Geometry check sheet. Reference: the model listing, model coordinates, mm. A direction names the side the tool comes from. Give positions to 0.01 mm unless a question says otherwise; leave off trailing zeros. Loops run counter-clockwise (first coordinate to the right, second up) from the corner with the lowest first, then second, coordinate; pieces in that order, holes last. Notation, with made-up numbers: (2.25, 52) -> (28.25, 52) arc R22 ccw to (28.25, 87) -> close; hole circle Ø3 at (-35.5, -4). An arc over 180 degrees is marked (long way). Write item = value, one per line.
```python
from build123d import *

# Parameters (mm, degrees)
SKETCH_1_W                 = 240
SKETCH_1_H                 = 100
EXTRUDE_1_DEPTH            = 6
SKETCH_2_R                 = 1.55
CUT_EXTRUDE_1_DEPTH        = 261.069221555
SKETCH_3_W                 = 60
SKETCH_3_H                 = 15
CUT_EXTRUDE_2_DEPTH        = 261.069221555
SKETCH_4_W                 = 30
SKETCH_4_H                 = 80
CUT_EXTRUDE_3_DEPTH        = 261.069221555
SKETCH_5_R                 = 3
CUT_EXTRUDE_4_DEPTH        = 3
EXTRUDE_2_DEPTH            = 240
EXTRUDE_3_DEPTH            = 5
PATTERN_LINEAR_5_COUNT     = 6
PATTERN_LINEAR_5_PITCH     = 20
PATTERN_LINEAR_5_COL_COUNT = 6
PATTERN_LINEAR_5_COL_PITCH = 20
FILLET_5_R                 = 5


with BuildPart() as part:
    # 草图1 → 凸台-拉伸1 (new body)
    with BuildSketch(Plane(origin=(0, 0, 0), x_dir=(0, 0, -1), z_dir=(1, 0, 0))):
        with Locations((120, -50)):
            Rectangle(SKETCH_1_W, SKETCH_1_H)
    extrude(amount=EXTRUDE_1_DEPTH)

    # 草图2 → 切除-拉伸1 (cut, through all)
    with BuildSketch(Plane(origin=(6, 0, 0), x_dir=(0, 0, -1), z_dir=(1, 0, 0))):
        with Locations((8, -54)):
            Circle(SKETCH_2_R)
        with Locations((45, -80)):
            Circle(SKETCH_2_R)
        with Locations((45, -54)):
            Circle(SKETCH_2_R)
        with Locations((8, -80)):
            Circle(SKETCH_2_R)
        with Locations(Location((232, -80, 0), (0, 0, 180))):
            Circle(SKETCH_2_R)
        with Locations(Location((195, -54, 0), (0, 0, 180))):
            Circle(SKETCH_2_R)
        with Locations(Location((195, -80, 0), (0, 0, 180))):
            Circle(SKETCH_2_R)
        with Locations(Location((232, -54, 0), (0, 0, 180))):
            Circle(SKETCH_2_R)
    extrude(amount=-CUT_EXTRUDE_1_DEPTH, mode=Mode.SUBTRACT)

    # 草图3 → 切除-拉伸2 (cut, through all)
    with BuildSketch(Plane(origin=(6, 0, 0), x_dir=(0, 0, -1), z_dir=(1, 0, 0))):
        with Locations((40, -27.5)):
            Rectangle(SKETCH_3_W, SKETCH_3_H)
        with Locations((200, -27.5)):
            Rectangle(SKETCH_3_W, SKETCH_3_H)
    extrude(amount=-CUT_EXTRUDE_2_DEPTH, mode=Mode.SUBTRACT)

    # 草图4 → 切除-拉伸3 (cut, through all)
    with BuildSketch(Plane(origin=(6, 0, 0), x_dir=(0, 0, -1), z_dir=(1, 0, 0))):
        with Locations((100, -50)):
            Rectangle(SKETCH_4_W, SKETCH_4_H)
        with Locations((140, -50)):
            Rectangle(SKETCH_4_W, SKETCH_4_H)
    extrude(amount=-CUT_EXTRUDE_3_DEPTH, mode=Mode.SUBTRACT)

    # 草图5 → 切除-拉伸4 (cut)
    with BuildSketch(Plane.ZY):
        with Locations((-195, -80)):
            Circle(SKETCH_5_R)
        with Locations((-232, -80)):
            Circle(SKETCH_5_R)
        with Locations((-195, -54)):
            Circle(SKETCH_5_R)
        with Locations((-232, -54)):
            Circle(SKETCH_5_R)
        with Locations((-45, -80)):
            Circle(SKETCH_5_R)
        with Locations((-8, -80)):
            Circle(SKETCH_5_R)
        with Locations((-8, -54)):
            Circle(SKETCH_5_R)
        with Locations((-45, -54)):
            Circle(SKETCH_5_R)
    extrude(amount=-CUT_EXTRUDE_4_DEPTH, mode=Mode.SUBTRACT)

    # 草图6 → 凸台-拉伸2 (add)
    with BuildSketch(Plane.XY):
        Polygon((6, 0), (0, 0), (0, 10.392304845), align=None)
    extrude(amount=-EXTRUDE_2_DEPTH)

    # 草图7 → 凸台-拉伸3 (add)
    with BuildSketch(Plane.XY.offset(-117.5)):
        Polygon((0, 10.392304845), (0, 15.392304845), (8, 1.535898385), (8, -8), (6, -8), (6, 0), align=None)
    extrude_3 = extrude(amount=-EXTRUDE_3_DEPTH)

    # 阵列(线性)5: 凸台-拉伸3 ×6
    with Locations(*[(0, 0, i * PATTERN_LINEAR_5_PITCH) for i in range(1, PATTERN_LINEAR_5_COUNT)]):
        add(extrude_3)

    # 阵列(线性)5 col: 凸台-拉伸3 ×6
    with Locations(*[(0, 0, -i * PATTERN_LINEAR_5_COL_PITCH) for i in range(1, PATTERN_LINEAR_5_COL_COUNT)]):
        add(extrude_3)

    # 圆角5
    fillet_5_edges = [part.edges().sort_by_distance(p)[0] for p in [
        (8, 1.535898385, -120),
        (8, 1.535898385, -140),
        (8, 1.535898385, -160),
        (8, 1.535898385, -180),
        (8, 1.535898385, -200),
        (8, 1.535898385, -220),
        (8, 1.535898385, -100),
        (8, 1.535898385, -80),
        (8, 1.535898385, -60),
        (8, 1.535898385, -40),
        (8, 1.535898385, -20),
    ]]
    fillet(fillet_5_edges, radius=FILLET_5_R)


solid = part.part
```
Item 1: Gauge pin test, flat ends, axial feed: pin 1 (2 mm diameter, centred on y = -29.5, z = -68, fed in from -X); pin 2 (1.5 mm diameter, centred on y = -79, z = -179.5, fed in from +X); pin 3 (4 mm diameter, centred on x = 5, y = 8, fed in from -Z); pin 4 (4 mm diameter, centred on x = 3, z = -165.5, fed in from +Y). Record the tip position at first contact, or that the pin passes through.
Answer:
pin_1 = through
pin_2 = 6
pin_3 = -222.5
pin_4 = 8.66
Item 2: Tool access check on faces 1 (the flat face through (3, -35, -40)), 2 (the flat face through (5, 4, -137.5)), 3 (the flat face through (3, -55.3, -6.7)). Record the directions out of +Z, -Z, +X, -X, +Y, -Y that give a thin tool (end or side, any length) a straight path to the whole face; none if there is none.
Answer:
face_1 = +X, -X
face_2 = +X, +Y
face_3 = -X
Item 3: Section check C-C, the plane x = 1.75. Give the number of separate pieces and of enclosed holes in the cut face, plus the area to 3 significant figures.
Answer:
separate_pieces = 1
enclosed_holes = 12
area = 19,200 mm^2
Item 4: Thickness scan on L1, parallel to Y at x = 4.45, z = -195; L2, parallel to Z at x = 1.5, y = -27; L3, parallel to Y at x = 4.15, z = -8. Record the ranges inside material, lowest first. Write a range as [from, to].
Answer:
L1 = [-100, -81.55], [-78.45, -55.55], [-52.45, -35], [-20, 2.68]
L2 = [-240, -230], [-170, -155], [-125, -115], [-85, -70], [-10, 0]
L3 = [-100, -81.55], [-78.45, -55.55], [-52.45, 3.2]
Item 5: Section check B-B, the plane z = -134.5. Record the cut outline in (x, y), plus the area to 3 significant figures.
Answer:
outline = (0, -100) -> (6, -100) -> (6, -90) -> (0, -90) -> close; (0, -10) -> (6, -10) -> (6, 0) -> (0, 10.39) -> close
area = 151 mm^2
Item 6: Draft check along Y on faces 4 (the flat face through (5, 4, -22.5)), 5 (the flat face through (3, -51, -155)), 6 (the flat face through (2.958, 5.269, -231.128)). Enter one of: +Y half, -Y half, draft (parallel to the pull), parting line (faces both ways), or undercut.
Answer:
face_4 = draft
face_5 = undercut
face_6 = +Y half
Item 7: Section check A-A, the plane z = -28.5. Record the cut outline in (x, y), plus the area to 3 significant figures.
Answer:
outline = (0, -100) -> (6, -100) -> (6, -35) -> (0, -35) -> close; (0, -20) -> (6, -20) -> (6, 0) -> (0, 10.39) -> close
area = 541 mm^2
